Model file for the job. Use its own axes, mm. A direction names the side the tool comes from. Round coordinates to 2 decimals unless told otherwise and drop trailing zeros. Order: outer loops, then holes, each group sorted by start corner. A loop starts at its lowest first (then second) coordinate and runs counter-clockwise, first axis right, second up. Notation, with made-up numbers: (23.25, 25.5) -> (63.25, 25.5) arc R19 ccw to (63.25, 49.5) -> close; hole circle Ø3 at (19.25, -9.5). An arc over 180 degrees is marked (long way). Answer as CSV lines item,"result".
```python
from build123d import *

# Parameters (mm, degrees)
SKETCH1_W           = 40
SKETCH1_H           = 60
BOSS_EXTRUDE1_DEPTH = 12.5
SKETCH4_W           = 4
SKETCH4_H           = 60
CUT_EXTRUDE1_DEPTH  = 10
CUT_EXTRUDE2_DEPTH  = 4
FILLET1_R           = 20
SKETCH6_W           = 20
SKETCH6_H           = 25
BOSS_EXTRUDE2_DEPTH = 10
FILLET2_SIZE        = 15
FILLET2_SIZE_2      = 20


with BuildPart() as part:
    # Sketch1 → Boss-Extrude1 (new, symmetric)
    with BuildSketch(Plane.XY):
        Rectangle(SKETCH1_W, SKETCH1_H)
    extrude(amount=BOSS_EXTRUDE1_DEPTH, both=True)

    # Sketch3 → Cut-Revolve1 (revolve, cut)
    with BuildSketch(Plane(origin=(0, 0, 0), x_dir=(0, 0, -1), z_dir=(1, 0, 0)), mode=Mode.PRIVATE) as cut_revolve1_sk:
        Polygon((-12.5, -8.157480559), (-7.5, -8.157480559), (-7.5, -4.169784019), (7.5, -4.169784019), (7.5, -8.157480559), (12.5, -8.157480559), (12.5, 0), (-12.5, 0), align=None)
    revolve(cut_revolve1_sk.sketch.rotate(Axis((0, 0, 19.169416837), (0, 0, -1)), 270), axis=Axis((0, 0, 19.169416837), (0, 0, -1)), mode=Mode.SUBTRACT)

    # Sketch4 → Cut-Extrude1 (cut)
    with BuildSketch(Plane.ZY.offset(20)):
        with Locations((-0.695939916, 0)):
            Rectangle(SKETCH4_W, SKETCH4_H)
    extrude(amount=-CUT_EXTRUDE1_DEPTH, mode=Mode.SUBTRACT)

    # Sketch5 → Cut-Extrude2 (cut)
    with BuildSketch(Plane.XY.offset(-12.5)):
        Polygon((0, -5.5), (-20, 1.779404685), (-20, 3.184119345), (0, -4.09528534), align=None)
    extrude(amount=CUT_EXTRUDE2_DEPTH, mode=Mode.SUBTRACT)

    # Fillet1
    fillet1_edges = [part.edges().sort_by_distance(p)[0] for p in [
        (20, 30, 0),
        (20, -30, 0),
    ]]
    fillet(fillet1_edges, radius=FILLET1_R)

    # Sketch6 → Boss-Extrude2 (add)
    with BuildSketch(Plane(origin=(0, -30, 0), x_dir=(1, 0, 0), z_dir=(0, 1, 0))):
        with Locations((-10, 0)):
            Rectangle(SKETCH6_W, SKETCH6_H)
    extrude(amount=-BOSS_EXTRUDE2_DEPTH)

    # Fillet2
    # an asymmetric fillet: 20, 15 mm, written as the material it takes off along each edge
    with BuildSketch(Plane(origin=(-20, -40, -62.5), x_dir=(1, 0, 0), z_dir=(0, 0, 1))) as fillet2_piece_1:
        with BuildLine():
            Bezier((FILLET2_SIZE, 0), (0, 0), (0, FILLET2_SIZE_2), weights=[1, 0.707106781, 1])
            Line((0, FILLET2_SIZE_2), (0, 0))
            Line((0, 0), (FILLET2_SIZE, 0))
        make_face()
    extrude(amount=125, mode=Mode.SUBTRACT)


solid = part.part
```
Q1. Saw through at A-A (y = 0). Write the cut outline in (x, z), plus the area to 3 significant figures.
Checks:
outline,"(-20, -12.5) -> (-15.11, -12.5) -> (-15.11, -8.5) -> (-11.25, -8.5) -> (-11.25, -12.5) -> (-8.16, -12.5) -> (-8.16, -7.5) -> (-4.17, -7.5) -> (-4.17, 7.5) -> (-8.16, 7.5) -> (-8.16, 12.5) -> (-20, 12.5) -> (-20, 1.3) -> (-10, 1.3) -> (-10, -2.7) -> (-20, -2.7) -> close; (4.17, -7.5) -> (8.16, -7.5) -> (8.16, -12.5) -> (20, -12.5) -> (20, 12.5) -> (8.16, 12.5) -> (8.16, 7.5) -> (4.17, 7.5) -> close"
area,"656 mm²"
Q2. Mould opens along Y. For faces 5 (the flat face through (-9, -5, 12.5)), 6 (the flat face through (-14, 0, -8.5)), 7 (the cylindrical face through (13.986, -24.297, 0.175)) say: +Y half, -Y half, draft (parallel to the pull), parting line (faces both ways), or undercut.
Checks:
face 5,"draft"
face 6,"undercut"
face 7,"-Y half"
Q3. Saw through at B-B (y = 23.5). Write the cut outline in (x, z).
Checks:
outline,"(-20, -12.5) -> (14.76, -12.5) -> (14.76, 12.5) -> (-20, 12.5) -> (-20, 1.3) -> (-10, 1.3) -> (-10, -2.7) -> (-20, -2.7) -> close"
Q4. Wall check: L1, parallel to Z at x = -11, y = -16; L2, parallel to Z at x = -1, y = 7; L3, parallel to Y at x = -3, z = 8.5. Give the ranges that are in metal, low to high. Write a range as [from, to].
Checks:
L1,"[-12.5, -2.7], [1.3, 12.5]"
L2,"[-7.5, 7.5]"
L3,"[-40, -7.59], [7.59, 30]"
Q5. Saw through at D-D (y = -11.5). Write the cut outline in (x, z), plus the area to 3 significant figures.
Checks:
outline,"(-20, -12.5) -> (19.94, -12.5) -> (19.94, 12.5) -> (-20, 12.5) -> (-20, 1.3) -> (-10, 1.3) -> (-10, -2.7) -> (-20, -2.7) -> close"
area,"959 mm²"
Q6. Tool access for faces 1 (the flat face through (0, -35, 0)), 2 (the flat face through (-14, -30, -1)), 3 (the flat face through (4, -2, -7.5)), 4 (the cylindrical face through (7.535, 3.124, 9.965)): list every direction of +Z, -Z, +X, -X, +Y, -Y with a clear straight run to the whole face (end or side of a thin tool).
Checks:
face 1,"+Z, -Z, +X, -Y"
face 2,"-X, +Y"
face 3,"-Z"
face 4,"+Z"
Q7. Saw through at C-C (x = 15). Write the cut outline in (y, z), plus the area to 3 significant figures.
Checks:
outline,"(-23.23, -12.5) -> (23.23, -12.5) -> (23.23, 12.5) -> (-23.23, 12.5) -> close"
area,"1,160 mm²"
Q8. Flat gauge pins, fed straight in: pin 1 (5 mm diameter, centred on y = -35.5, z = 2, fed in from +X); pin 2 (13 mm diameter, centred on x = 0, y = 0, fed in from -Z); pin 3 (8 mm diameter, centred on x = -1, y = -3, fed in from +Z). Where does each tip first touch, or does it go through?
Checks:
pin 1,"x = 0"
pin 2,"z = -7.5"
pin 3,"z = 7.5"
